Part model, mm, in its own coordinate system. Face numbers are marked on the shaded views. A direction names the side the tool comes from. Round coordinates to 2 decimals unless told otherwise and drop trailing zeros. Loops run counter-clockwise (first coordinate to the right, second up) from the corner with the lowest first, then second, coordinate; pieces in that order, holes last.
from build123d import *

# Parameters (mm, degrees)
BOSS_EXTRU_1_DEPTH      = 2.4
BOSS_EXTRU_2_DEPTH      = 6
ESQUISSE2_R             = 0.78
ENL_V_MAT_EXTRU_1_DEPTH = 51.646782553
ESQUISSE3_R             = 3.6
ENL_V_MAT_EXTRU_2_DEPTH = 0.6
ESQUISSE4_R             = 3
ENL_V_MAT_EXTRU_3_DEPTH = 3.6
ESQUISSE5_R             = 1.2
ENL_V_MAT_EXTRU_4_DEPTH = 3.6


with BuildPart() as part:
    # Esquisse1 → Boss.-Extru.1 (new body)
    with BuildSketch(Plane.XY):
        with BuildLine():
            Line((-50.290124109, 0), (-28.762124109, 0))
            ThreePointArc((-28.762124109, 0), (-27.607292966, 3.122938361), (-24.698480773, 4.743182356))
            Line((-24.698480773, 4.743182356), (-47.290124109, 3))
            ThreePointArc((-47.290124109, 3), (-49.411444453, 2.121320344), (-50.290124109, 0))
        make_face()
        with BuildLine():
            ThreePointArc((-24.698480773, -4.743182356), (-27.607292966, -3.122938361), (-28.762124109, 0))
            Line((-28.762124109, 0), (-50.290124109, 0))
            ThreePointArc((-50.290124109, 0), (-49.411444453, -2.121320344), (-47.290124109, -3))
            Line((-47.290124109, -3), (-24.698480773, -4.743182356))
        make_face()
    extrude(amount=BOSS_EXTRU_1_DEPTH)

    # Esquisse1_3 → Boss.-Extru.2 (add)
    with BuildSketch(Plane.XY):
        with BuildLine():
            Line((-28.762124109, 0), (-19.162124109, 0))
            ThreePointArc((-19.162124109, 0), (-20.56801156, 3.39411255), (-23.962124109, 4.8))
            Line((-23.962124109, 4.8), (-24.698480773, 4.743182356))
            ThreePointArc((-24.698480773, 4.743182356), (-27.607292966, 3.122938361), (-28.762124109, 0))
        make_face()
        with BuildLine():
            ThreePointArc((-23.962124109, -4.8), (-20.56801156, -3.39411255), (-19.162124109, 0))
            Line((-19.162124109, 0), (-28.762124109, 0))
            ThreePointArc((-28.762124109, 0), (-27.607292966, -3.122938361), (-24.698480773, -4.743182356))
            Line((-24.698480773, -4.743182356), (-23.962124109, -4.8))
        make_face()
    extrude(amount=BOSS_EXTRU_2_DEPTH)

    # Esquisse2 → Enl_v. mat.-Extru.1 (cut, through all)
    with BuildSketch(Plane.XY.offset(2.4)):
        with Locations((-47.481401961, 0)):
            Circle(ESQUISSE2_R)
        with Locations((-45.081401961, 0)):
            Circle(ESQUISSE2_R)
        with Locations((-42.681401961, 0)):
            Circle(ESQUISSE2_R)
        with Locations((-40.281401961, 0)):
            Circle(ESQUISSE2_R)
    extrude(amount=-ENL_V_MAT_EXTRU_1_DEPTH, mode=Mode.SUBTRACT)

    # Esquisse3 → Enl_v. mat.-Extru.2 (cut)
    with BuildSketch(Plane(origin=(0, 0, 0), x_dir=(-1, 0, 0), z_dir=(0, 0, -1))):
        with Locations((23.962124109, 0)):
            Circle(ESQUISSE3_R)
    extrude(amount=-ENL_V_MAT_EXTRU_2_DEPTH, mode=Mode.SUBTRACT)

    # Esquisse4 → Enl_v. mat.-Extru.3 (cut)
    with BuildSketch(Plane.XY.offset(6)):
        with Locations((-23.884137935, 0)):
            Circle(ESQUISSE4_R)
    extrude(amount=-ENL_V_MAT_EXTRU_3_DEPTH, mode=Mode.SUBTRACT)

    # Esquisse5 → Enl_v. mat.-Extru.4 (cut)
    with BuildSketch(Plane.XY.offset(2.4)):
        with Locations((-23.884137935, 0)):
            Circle(ESQUISSE5_R)
    extrude(amount=-ENL_V_MAT_EXTRU_4_DEPTH, mode=Mode.SUBTRACT)


solid = part.part
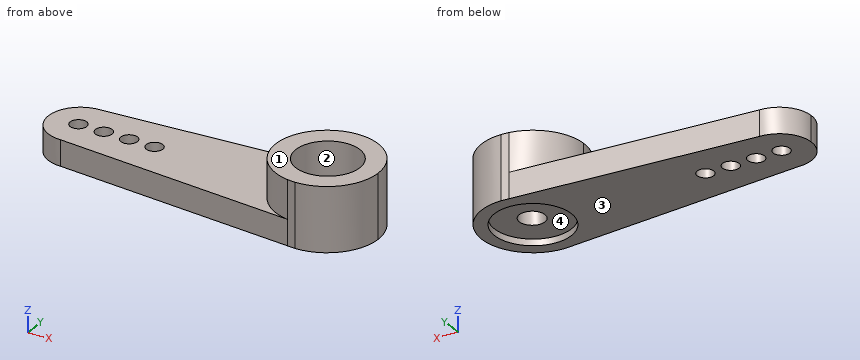
1) Slice it at D-D, the plane x = -25.5. Give the cut face in (y, z), then the cut area to 3 significant figures.
Values:
outline: (-4.68, 0) - (-3.25, 0) - (-3.25, 0.6) - (3.25, 0.6) - (3.25, 0) - (4.68, 0) - (4.68, 2.4) - (4.55, 2.4) - (4.55, 6) - (2.53, 6) - (2.53, 2.4) - (-2.53, 2.4) - (-2.53, 6) - (-4.55, 6) - (-4.55, 2.4) - (-4.68, 2.4) - close
area: 33.1 mm2
2) Slice it at C-C, the plane y = -1.5. Give the cut face in (x, z).
Values:
outline: (-49.89, 0) - (-27.23, 0) - (-27.23, 0.6) - (-20.69, 0.6) - (-20.69, 0) - (-19.4, 0) - (-19.4, 6) - (-21.29, 6) - (-21.29, 2.4) - (-26.48, 2.4) - (-26.48, 6) - (-28.52, 6) - (-28.52, 2.4) - (-49.89, 2.4) - close
3) Tool access for the marked faces 1 and 2: list every direction of +Z, -Z, +X, -X, +Y, -Y with a clear straight run to the whole face (end or side of a thin tool).
Values:
face 1: +Z, +X, -X, +Y, -Y
face 2: +Z
4) Mould opens along X. For the marked faces 3 and 4 say: released by +X, released by -X, zero draft, split by the parting line, or undercut.
Values:
face 3: zero draft
face 4: undercut
5) Wall check: line 1 along X through (y, z) = (-0.25, 2); line 2 along Y through (x, z) = (-24, 4.5); line 3 along Z through (x, y) = (-27, -1.5). Give the ranges that are in metal, low to high.
Values:
line 1: x = -50.28 to -48.22, -46.74 to -45.82, -44.34 to -43.42, -41.94 to -41.02, -39.54 to -25.06, -22.71 to -19.17
line 2: y = -4.8 to -3, 3 to 4.8
line 3: z = 0.6 to 6
6) Slice it at A-A, the plane z = 1.4. Give the cut face in (x, y).
Values:
outline: (-47.29, -3) - (-23.96, -4.8) arc R4.8 ccw to (-23.96, 4.8) - (-47.29, 3) arc R3 ccw to start; hole circle Ø1.56 at (-47.48, 0); hole circle Ø1.56 at (-45.08, 0); hole circle Ø1.56 at (-42.68, 0); hole circle Ø1.56 at (-40.28, 0); hole circle Ø2.4 at (-23.88, 0)
7) Slice it at B-B, the plane z = 4.9. Give the cut face in (x, y).
Values:
outline: (-24.7, -4.74) - (-23.96, -4.8) arc R4.8 ccw to (-23.96, 4.8) - (-24.7, 4.74) arc R4.8 ccw to start; hole circle Ø6 at (-23.88, 0)
8) Drop flat-ended pins along their axis: pin 1 Ø1.8 at (x, y) = (-24, 1) entering from +Z; pin 2 Ø1.5 at (y, z) = (2, 2) entering from -X; pin 3 Ø3.5 at (x, y) = (-23.88, 0) entering from -Z. Give the stop position or say it passes through.
Values:
pin 1: stops at z = 2.4
pin 2: stops at x = -50.02
pin 3: stops at z = 0.6
